from build123d import *

# Parameters (mm, degrees)
BOSS_EXTRUDE1_DEPTH = 10
SKETCH3_R           = 73
SKETCH2_R           = 52.5
FILLET3_R           = 5
FILLET4_R           = 20
SHELL4_T            = -2
BOSS_EXTRUDE3_START = 8
BOSS_EXTRUDE3_DEPTH = 8
SKETCH16_R          = 2
CUT_EXTRUDE8_DEPTH  = 9
SKETCH5_R           = 54.5
SKETCH5_R_2         = 52.5
BOSS_EXTRUDE2_DEPTH = 60
SKETCH9_R           = 112.367107934
CUT_EXTRUDE5_DEPTH  = 60
SKETCH10_R          = 91.913425111
CUT_EXTRUDE6_DEPTH  = 10
SKETCH11_R          = 79.181330982
CUT_EXTRUDE7_DEPTH  = 10
FILLET5_R           = 5
FILLET6_R           = 5
FILLET7_R           = 3
FILLET8_R           = 5
FILLET9_R           = 2
FILLET10_R          = 5


with BuildPart() as part:
    # Sketch1 → Boss-Extrude1 (new body)
    with BuildSketch(Plane.XY):
        with BuildLine():
            Line((100, 99.277863028), (100, 19.277863028))
            Line((100, 19.277863028), (0, -110.722136972))
            Line((0, -110.722136972), (-100, 19.277863028))
            Line((-100, 19.277863028), (-100, 99.277863028))
            ThreePointArc((-100, 99.277863028), (0, 109.277863028), (100, 99.277863028))
        make_face()
    extrude(amount=BOSS_EXTRUDE1_DEPTH)

    # Sketch3 → Cut-Loft1 section 0
    with BuildSketch(Plane.XY.offset(10)):
        with Locations((0, 29.277863028)):
            Circle(SKETCH3_R)
    # Sketch2 → Cut-Loft1 section 1
    with BuildSketch(Plane.XY):
        with Locations((0, 29.277863028)):
            Circle(SKETCH2_R)
    loft(mode=Mode.SUBTRACT)

    # Fillet3
    fillet3_edges = [part.edges().sort_by_distance(p)[0] for p in [
        (0, -110.722136972, 5),
    ]]
    fillet(fillet3_edges, radius=FILLET3_R)

    # Fillet4
    fillet4_edges = [part.edges().sort_by_distance(p)[0] for p in [
        (100, 19.277863028, 5),
        (-100, 19.277863028, 5),
    ]]
    fillet(fillet4_edges, radius=FILLET4_R)

    # Shell4
    shell4_openings = [part.faces().sort_by_distance(p)[0] for p in [
        (47.569868433, -44.043588356, 0),
    ]]
    offset(amount=SHELL4_T, openings=shell4_openings, kind=Kind.INTERSECTION)

    # Sketch12 → Boss-Extrude3 (add)
    with BuildSketch(Plane(origin=(0, 0, 8), x_dir=(-1, 0, 0), z_dir=(0, 0, -1)).offset(BOSS_EXTRUDE3_START)):
        with BuildLine():
            Line((-9.169512185, -95.521527238), (9.169512185, -95.521527238))
            Line((9.169512185, -95.521527238), (2.377871967, -104.350659521))
            ThreePointArc((2.377871967, -104.350659521), (0, -105.521527238), (-2.377871967, -104.350659521))
            Line((-2.377871967, -104.350659521), (-9.169512185, -95.521527238))
        make_face()
        with BuildLine():
            Line((98, 87.63878568), (98, 97.63878568))
            ThreePointArc((98, 97.63878568), (93.090974034, 98.588565475), (88.172749454, 99.48950087))
            ThreePointArc((88.172749454, 99.48950087), (90.302365562, 91.255493109), (98, 87.63878568))
        make_face()
        with BuildLine():
            Line((-98, 97.63878568), (-98, 87.63878568))
            ThreePointArc((-98, 87.63878568), (-90.302365562, 91.255493109), (-88.172749454, 99.48950087))
            ThreePointArc((-88.172749454, 99.48950087), (-93.090974034, 98.588565475), (-98, 97.63878568))
        make_face()
    extrude(amount=-BOSS_EXTRUDE3_DEPTH)

    # Sketch16 → Cut-Extrude8 (cut, symmetric)
    with BuildSketch(Plane(origin=(0, 0, 8), x_dir=(-1, 0, 0), z_dir=(0, 0, -1))):
        with Locations((0, -99.521527238)):
            Circle(SKETCH16_R)
        with Locations((-93, 94.13878568)):
            Circle(SKETCH16_R)
        with Locations((93, 94.13878568)):
            Circle(SKETCH16_R)
    extrude(amount=CUT_EXTRUDE8_DEPTH, both=True, mode=Mode.SUBTRACT)

    # Sketch5 → Boss-Extrude2 (add)
    with BuildSketch(Plane(origin=(0, 0, 0), x_dir=(-1, 0, 0), z_dir=(0, 0, -1))):
        with Locations(Location((0, 29.277863028, 0), (0, 0, 180))):
            Circle(SKETCH5_R)
        with Locations(Location((0, 29.277863028, 0), (0, 0, 180))):
            Circle(SKETCH5_R_2, mode=Mode.SUBTRACT)
    extrude(amount=BOSS_EXTRUDE2_DEPTH)

    # Sketch9 → Cut-Extrude5 (cut)
    with BuildSketch(Plane(origin=(0, -4.696341029, -10.071335838), x_dir=(-1, 0, 0), z_dir=(0, -0.42261826174070327, -0.9063077870366482))):
        with Locations((0, 89.719397921)):
            Circle(SKETCH9_R)
    extrude(amount=CUT_EXTRUDE5_DEPTH, mode=Mode.SUBTRACT)

    # Sketch10 → Cut-Extrude6 (cut)
    with BuildSketch(Plane(origin=(0, -4.030519152, -9.495308079), x_dir=(-1, 0, 0), z_dir=(0, -0.39073112848928093, -0.9205048534524374))):
        with Locations((0, 68.891691178)):
            Circle(SKETCH10_R)
    extrude(amount=CUT_EXTRUDE6_DEPTH, mode=Mode.SUBTRACT)

    # Sketch11 → Cut-Extrude7 (cut)
    with BuildSketch(Plane(origin=(0, -3.111126453, -8.547749678), x_dir=(-1, 0, 0), z_dir=(0, -0.34202014332567576, -0.9396926207859059))):
        with Locations((0, 55.651285061)):
            Circle(SKETCH11_R)
    extrude(amount=CUT_EXTRUDE7_DEPTH, mode=Mode.SUBTRACT)

    # Fillet5
    fillet5_edges = [part.edges().sort_by_distance(p)[0] for p in [
        (100, 99.277863028, 5),
    ]]
    fillet(fillet5_edges, radius=FILLET5_R)

    # Fillet6
    fillet6_edges = [part.edges().sort_by_distance(p)[0] for p in [
        (-100, 99.277863028, 5),
    ]]
    fillet(fillet6_edges, radius=FILLET6_R)

    # Fillet7
    fillet7_edges = [part.edges().sort_by_distance(p)[0] for p in [
        (0, 109.277863028, 10),
        (98.856812155, 98.351888702, 10),
        (-100, 60.625105075, 10),
        (-98.856812155, 98.351888702, 10),
        (49.907799864, -45.841997149, 10),
        (0, -107.521527238, 10),
        (100, 60.625105075, 10),
        (-49.907799864, -45.841997149, 10),
        (-98.934751063, 19.640177571, 10),
        (98.934751063, 19.640177571, 10),
    ]]
    fillet(fillet7_edges, radius=FILLET7_R)

    # Fillet8
    fillet8_edges = [part.edges().sort_by_distance(p)[0] for p in [
        (-73, 29.277863028, 10),
    ]]
    fillet(fillet8_edges, radius=FILLET8_R)

    # Fillet9
    fillet9_edges = [part.edges().sort_by_distance(p)[0] for p in [
        (-54.5, 29.277863028, 0),
    ]]
    fillet(fillet9_edges, radius=FILLET9_R)

    # Fillet10
    # the kernel refuses this fillet: 5 mm, written as the material it adds along each edge
    with BuildSketch(Plane(origin=(-80, 26.080301962, 8), x_dir=(-1, 0, 0), z_dir=(0, 1, 0))) as fillet10_piece_1:
        with BuildLine():
            CenterArc((18 - FILLET10_R, -FILLET10_R), FILLET10_R, 0, 90)
            Line((18, -FILLET10_R), (18 + FILLET10_R * 0.02, -FILLET10_R))
            Line((18 + FILLET10_R * 0.02, -FILLET10_R), (18 + FILLET10_R * 0.02, FILLET10_R * 0.02))
            Line((18 + FILLET10_R * 0.02, FILLET10_R * 0.02), (18 - FILLET10_R, FILLET10_R * 0.02))
            Line((18 - FILLET10_R, FILLET10_R * 0.02), (18 - FILLET10_R, 0))
        make_face()
    revolve(axis=Axis((-80, 26.080301962, 8), (0, 0, 1)), revolution_arc=37.568592029)
    with BuildSketch(Plane(origin=(-1.548127674, -105.429327102, 8), x_dir=(0.7926239891046, 0.6097107608496924, 0), z_dir=(-0.6097107608496926, 0.7926239891046001, 0))) as fillet10_piece_2_section:
        with BuildLine():
            CenterArc((FILLET10_R, FILLET10_R), FILLET10_R, 180, 90)
            Line((0, FILLET10_R), (-FILLET10_R * 0.02, FILLET10_R))
            Line((-FILLET10_R * 0.02, FILLET10_R), (-FILLET10_R * 0.02, -FILLET10_R * 0.02))
            Line((-FILLET10_R * 0.02, -FILLET10_R * 0.02), (FILLET10_R, -FILLET10_R * 0.02))
            Line((FILLET10_R, -FILLET10_R * 0.02), (FILLET10_R, 0))
        make_face()
    fillet10_piece_2 = extrude(amount=152.07063756, mode=Mode.PRIVATE)
    fillet10_piece_2 = split(fillet10_piece_2, bisect_by=Plane(origin=(-50.54915131, -95.521527238, 6.871784101), z_dir=(0, 1, 0)), keep=Keep.TOP, mode=Mode.PRIVATE)
    add(fillet10_piece_2)
    with BuildSketch(Plane(origin=(-98, 26.080301962, 8), x_dir=(1, 0, 0), z_dir=(0, 1, 0))) as fillet10_piece_3_section:
        with BuildLine():
            CenterArc((FILLET10_R, FILLET10_R), FILLET10_R, 180, 90)
            Line((0, FILLET10_R), (-FILLET10_R * 0.02, FILLET10_R))
            Line((-FILLET10_R * 0.02, FILLET10_R), (-FILLET10_R * 0.02, -FILLET10_R * 0.02))
            Line((-FILLET10_R * 0.02, -FILLET10_R * 0.02), (FILLET10_R, -FILLET10_R * 0.02))
            Line((FILLET10_R, -FILLET10_R * 0.02), (FILLET10_R, 0))
        make_face()
    fillet10_piece_3 = extrude(amount=74.058483718, mode=Mode.PRIVATE)
    fillet10_piece_3 = fillet10_piece_3 - Plane(origin=(-98, 97.63878568, 6.86971186), x_dir=(0.9827250545662549, 0.18507151895348808, 0), z_dir=(0, 0, -1)) * Cylinder(10, 169, mode=Mode.PRIVATE)
    add(fillet10_piece_3)
    with BuildSketch(Plane(origin=(0, -395.722136972, 8), x_dir=(-0.19970369332898327, 0.9798563337912163, 0), z_dir=(-0.9798563337912163, -0.19970369332898327, 0))) as fillet10_piece_4_section:
        with BuildLine():
            CenterArc((503 - FILLET10_R, FILLET10_R), FILLET10_R, 270, 90)
            Line((503, FILLET10_R), (503 + FILLET10_R * 0.02, FILLET10_R))
            Line((503 + FILLET10_R * 0.02, FILLET10_R), (503 + FILLET10_R * 0.02, -FILLET10_R * 0.02))
            Line((503 + FILLET10_R * 0.02, -FILLET10_R * 0.02), (503 - FILLET10_R, -FILLET10_R * 0.02))
            Line((503 - FILLET10_R, -FILLET10_R * 0.02), (503 - FILLET10_R, 0))
        make_face()
    fillet10_piece_4 = revolve(axis=Axis((0, -395.722136972, 8), (0, 0, -1)), revolution_arc=23.03926473, mode=Mode.PRIVATE)
    fillet10_piece_4 = fillet10_piece_4 - Plane(origin=(-98, 97.63878568, 6.609161961), x_dir=(0.9827250545662549, 0.18507151895348808, 0), z_dir=(0, 0, -1)) * Cylinder(10, 2013, mode=Mode.PRIVATE)
    fillet10_piece_4 = fillet10_piece_4 - Plane(origin=(98, 97.63878568, 6.609161961), x_dir=(0, -1, 0), z_dir=(0, 0, -1)) * Cylinder(10, 2013, mode=Mode.PRIVATE)
    add(fillet10_piece_4)


solid = part.part
Can you work these out from the model? Positions are in its coordinate system, mm. A direction names the side the tool comes from. Give positions to 0.01 mm unless a question says otherwise; leave off trailing zeros. Loops run counter-clockwise (first coordinate to the right, second up) from the corner with the lowest first, then second, coordinate; pieces in that order, holes last. Notation, with made-up numbers: M 4,62 L 36,62 A28 ccw 36,101 Z; hole C 48.25,25.5 d9. An arc over 180 degrees is marked long. One line per item, written item: value.
1) On a 3-axis mill with a long thin cutter (end or side, diameter ignored), from which of +Z, -Z, +X, -X, +Y, -Y can I reach the whole of each face in a straight line? I mean faces 1 (the face through (52.314, -39.434, 3.944)), 2 (the face through (48.55, -46.128, 9.145)). Say none if no direction works.
Geometry check:
face 1: -Z
face 2: +Z, +X, -Y
2) Please list where these lines run through material, in increasing order: line 1 (Y direction, x = -12.5, z = 2); line 2 (Y direction, x = 93, z = 7); line 3 (Y direction, x = -93, z = 4).
Geometry check:
line 1: y = -94.47 to -91.19, -30.59 to -25.92, 84.48 to 89.15, 107.12 to 109.12
line 2: y = 10.18 to 13.46, 88.98 to 92.14, 96.14 to 100.64
line 3: y = 10.18 to 13.62, 88.98 to 92.14, 96.14 to 100.64
3) I'm going to push flat-ended pins straight in: pin 1 (4 mm diameter, centred on y = 19, z = -0.5, fed in from -X); pin 2 (1.5 mm diameter, centred on y = 79, z = -21.5, fed in from -X); pin 3 (6 mm diameter, centred on x = 4, z = -13.5, fed in from +Y). Where does each tip first touch, or does it pass through?
Geometry check:
pin 1: stops at x = -99.33
pin 2: stops at x = -23.92
pin 3: stops at y = 83.77
4) Thinking about a two-plate mould opening in Y: for faces 3 (the face through (-11.38, 80.53, -15.21)), 4 (the face through (-1.241, 107.276, 1.479)), 5 (the face through (0.06, -107.52, 3.55)), 6 (the face through (66, -23, 0)), which applies, +Y half, -Y half, draft (parallel to the pull), parting line (faces both ways), or undercut?
Geometry check:
face 3: undercut
face 4: undercut
face 5: -Y half
face 6: draft
5) Imagine slicing it at B-B on z = -27.5. Write out the boundary of the cut face in (x, y), and give its area (3 significant figures).
Geometry check:
outline: M -50.82,48.96 L -48.67,48.96 A52.5 cw 48.67,48.96 L 50.82,48.96 A54.5 ccw Z
area: 256 mm²
6) Imagine slicing it at A-A on z = -12.5. Write out the boundary of the cut face in (x, y).
Geometry check:
outline: M -50.07,7.75 L -47.88,7.75 A52.5 cw long 47.88,7.75 L 50.07,7.75 A54.5 ccw long Z
